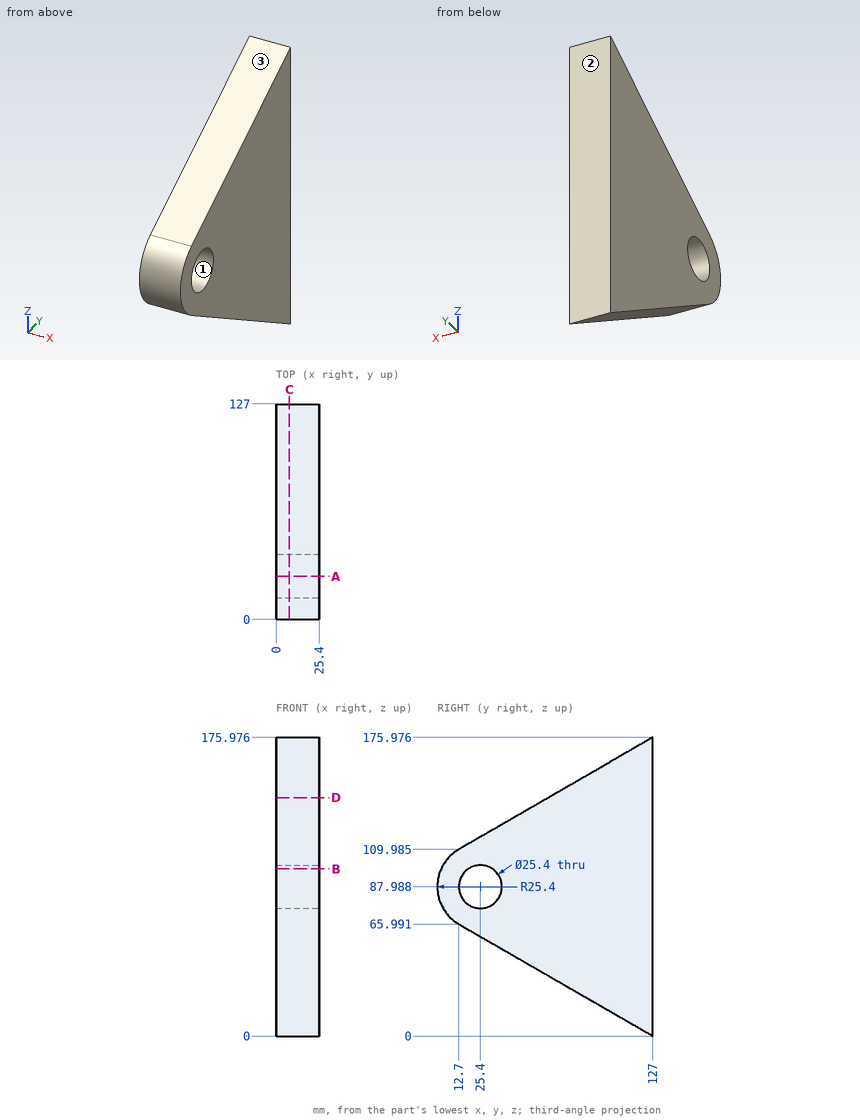
The drawing under review shows one solid part. Ordinate dimensions are in mm from its lowest x, y, z. Coordinates: 2 decimals unless noted, no trailing zeros. Order: outer loops, then holes, each group sorted by start corner. A loop starts at its lowest first (then second) coordinate and runs counter-clockwise, first axis right, second up. Notation, with made-up numbers: (-36.75, -18.75) -> (13.25, -18.75) arc R21 ccw to (13.25, -13.75) -> close; hole circle Ø2 at (-15.5, 83.5). An arc over 180 degrees is marked (long way). Answer in a Markdown table with one row per item.
(1) The part is to be moulded in two halves that separate along Z. For the marked faces 1, 2 and 3, say which applies: +Z half, -Z half, draft (parallel to the pull), parting line (faces both ways), or undercut.
Answers:
| item | result |
|---|---|
| face 1 | undercut |
| face 2 | draft |
| face 3 | +Z half |
(2) Consider section A-A (y = 25.4). Write out the cut boundary in (x, z).
Answers:
| item | result |
|---|---|
| outline | (0, 58.66) -> (25.4, 58.66) -> (25.4, 75.29) -> (0, 75.29) -> close; (0, 100.69) -> (25.4, 100.69) -> (25.4, 117.32) -> (0, 117.32) -> close |
(3) Consider section B-B (z = 98.5). Write out the cut boundary in (x, y).
Answers:
| item | result |
|---|---|
| outline | (0, 2.28) -> (25.4, 2.28) -> (25.4, 18.27) -> (0, 18.27) -> close; (0, 32.53) -> (25.4, 32.53) -> (25.4, 127) -> (0, 127) -> close |
(4) Consider section C-C (x = 7.75). Write out the cut boundary in (y, z) (1 decimal).
Answers:
| item | result |
|---|---|
| outline | (12.7, 66) -> (127, 0) -> (127, 176) -> (12.7, 110) arc R25.4 ccw to start; hole circle Ø25.4 at (25.4, 88) |
(5) Insertion check: pin 1 (3 mm diameter, centred on x = 16.5, z = 137.5, fed in from -Y); pin 2 (4 mm diameter, centred on x = 19, y = 34, fed in from -Z); pin 3 (4 mm diameter, centred on x = 5.5, y = 42, fed in from +Z). Each pin has a flat end and moves straight along its axis. Give the tip position at first contact, or say it passes through.
Answers:
| item | result |
|---|---|
| pin 1 | y = 57.76 |
| pin 2 | z = 52.54 |
| pin 3 | z = 128.06 |
(6) Wall thickness on line 1 along Y through (x, z) = (4, 88.5) (1 decimal); line 2 along Z through (x, y) = (17.75, 25.4); line 3 along Y through (x, z) = (13, 78.5): over which ranges is each line inside the solid? List them lowest first.
Answers:
| item | result |
|---|---|
| line 1 | 0 to 12.7, 38.1 to 127 |
| line 2 | 58.66 to 75.29, 100.69 to 117.32 |
| line 3 | 1.84 to 16.96, 33.84 to 127 |
(7) Consider section D-D (z = 140.5). Write out the cut boundary in (x, y).
Answers:
| item | result |
|---|---|
| outline | (0, 65.55) -> (25.4, 65.55) -> (25.4, 127) -> (0, 127) -> close |
